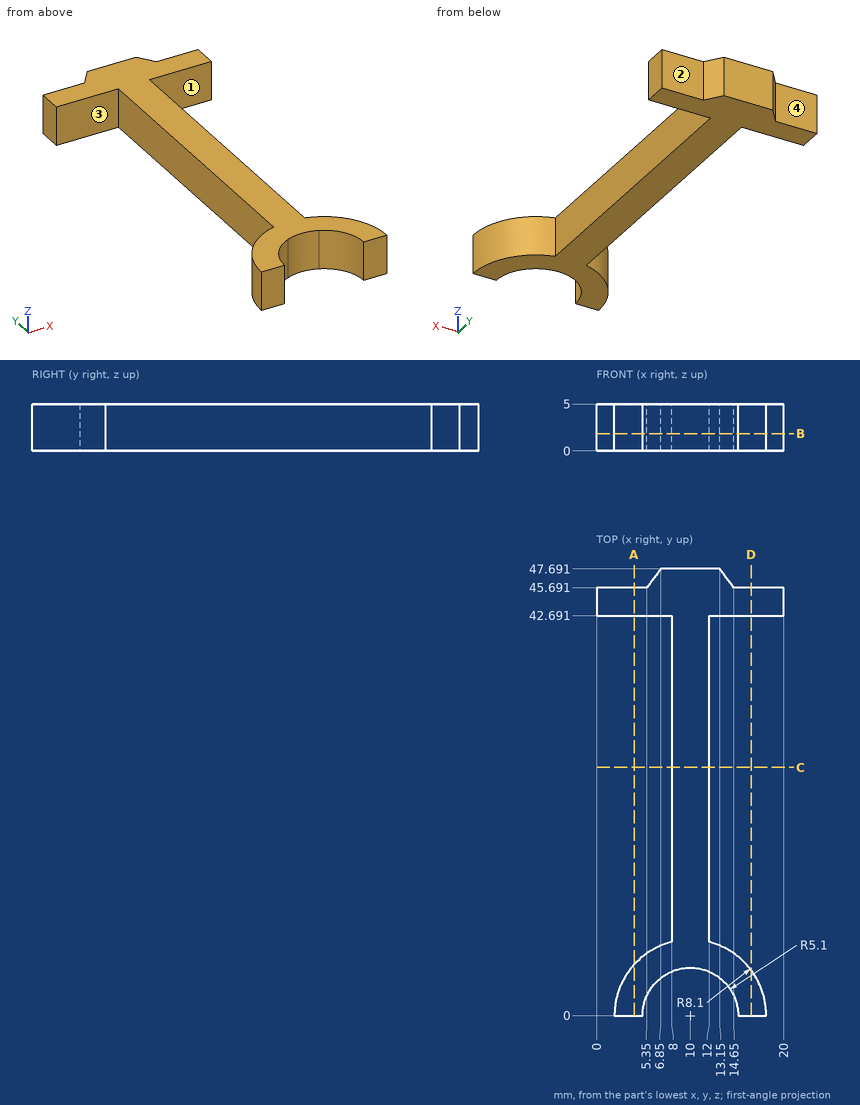
Source: three-view drawing plus pictorial views. Frame: mm from the lowest corner of the part. A direction names the side the tool comes from. Round coordinates to 2 decimals unless told otherwise and drop trailing zeros. Loops run counter-clockwise (first coordinate to the right, second up) from the corner with the lowest first, then second, coordinate; pieces in that order, holes last. Notation, with made-up numbers: M 6,33 L 50,33 A18 ccw 50,46 Z; hole C -9,85.25 d11. An arc over 180 degrees is marked long. Put each result on its own line as item: value. Start each with the question number.
(1) Section query A-A (x = 4). Return loops of the section in (y, z).
(2) Set-up query: the marked faces 1, 2, 3 and 4. Return all of +Z, -Z, +X, -X, +Y, -Y with unobstructed straight access to the full face (end or side cutting, diameter ignored); none if empty.
(3) Section query C-C (y = 26.5). Return loops of the section in (x, z), then the cut area to 3 significant figures.
(4) Section query B-B (z = 1.85). Return loops of the section in (x, y).
(5) Material intervals for line 1 along X through (y, z) = (17, 3.95); line 2 along X through (y, z) = (3, 1.15) (1 decimal); line 3 along Y through (x, z) = (17.25, 1.1) (1 decimal), sorted ascending. Write a range as [from, to].
(6) Section query D-D (x = 16.5). Return loops of the section in (y, z).
(7) Contact query for flat-ended pins moving along their axis: pin 1 Ø1.5 at (x, z) = (7.5, 1.5) entering from -Y; pin 2 Ø1 at (y, z) = (5, 2.5) entering from -X (1 decimal); pin 3 Ø3 at (x, y) = (15, 32) entering from -Z; pin 4 Ø2.5 at (x, z) = (3, 2) entering from +Y. Output: stop coordinate, or through.
Findings below:
1. outline: M 0,0 L 5.44,0 L 5.44,5 L 0,5 Z; M 42.69,0 L 45.69,0 L 45.69,5 L 42.69,5 Z
2. face 1: +Z, -Z, +X
2. face 2: +Z, -Z, +X, +Y
2. face 3: +Z, -Z, -X
2. face 4: +Z, -Z, -X, +Y
3. outline: M 8,0 L 12,0 L 12,5 L 8,5 Z
3. area: 20.0 mm2
4. outline: M 0,42.69 L 8,42.69 L 8,7.85 A8.1 ccw 1.9,0 L 4.9,0 A5.1 cw 8,4.69 A5.1 cw 12,4.69 A5.1 cw 15.1,0 L 18.1,0 A8.1 ccw 12,7.85 L 12,42.69 L 20,42.69 L 20,45.69 L 14.65,45.69 L 13.15,47.69 L 6.85,47.69 L 5.35,45.69 L 0,45.69 Z
5. line 1: x = [8, 12]
5. line 2: x = [2.5, 5.9], [14.1, 17.5]
5. line 3: y = [0, 3.6], [42.7, 45.7]
6. outline: M 0,0 L 4.83,0 L 4.83,5 L 0,5 Z; M 42.69,0 L 45.69,0 L 45.69,5 L 42.69,5 Z
7. pin 1: stops at y = 3.93
7. pin 2: stops at x = 3.3
7. pin 3: passes through
7. pin 4: stops at y = 45.69
